Model file for the job. Use its own axes, mm. A direction names the side the tool comes from. Coordinates: 2 decimals unless noted, no trailing zeros. Write each loop counter-clockwise with the first axis right and the second up, starting at its lowest first coordinate (ties: lowest second). Pieces come first, ordered by that corner, then holes. Notation, with made-up numbers: M 40,7.5 L 91,7.5 A18 cw 91,24.5 Z; hole C 51.5,65.25 d8. An arc over 180 degrees is marked long. Put each result on its own line as item: value. Start each with the question number.
Q1. Drill centre lines: line 1 along Y through (x, z) = (0, 4.25); line 2 along X through (y, z) = (-0.5, 3.25); line 3 along Y through (x, z) = (60.5, 2.5). Where is each one in solid material? Low to high.
Q2. Cut at B-B (x = 0). Write the cut outline in (y, z), then the cut area to 3 significant figures.
Q3. Cut at C-C (y = -1.5). Write the cut outline in (x, z), then the cut area to 3 significant figures.
Q4. Cut at D-D (y = -13). Write the cut outline in (x, z), then the cut area to 3 significant figures.
Q5. Pull direction Y, two halves, no side cores. Call faces 4 (the flat face through (-10, 0, 4)), 5 (the cylindrical face through (65.302, -2.069, 3.698)), 6 (the flat face through (33, 10, 4)), 7 (the flat face through (28, -10, 4)): pulls with the +Y half, pulls with the -Y half, needs draft (parallel to the pull), parting line crosses it, or undercut.
Q6. Which spindle directions (+Z, -Z, +X, -X, +Y, -Y) get a long thin tool onto all of the face, cutting with end or side? Do faces 1 (the flat face through (33, -1, 7.5)), 2 (the cylindrical face through (73.07, -39.48, 9.19)), 3 (the flat face through (68, -25, 4)). Say none if no direction does.
Q7. Cut at A-A (z = 2.5). Write the cut outline in (x, y), then the cut area to 3 significant figures.
Q8. Drop flat-ended pins along their axis: pin 1 (2 mm diameter, centred on x = 59.5, z = 8, fed in from -Y); pin 2 (6 mm diameter, centred on y = -19, z = 8, fed in from -X); pin 3 (20 mm diameter, centred on x = 31, y = -10.5, fed in from +Z). Give the stop position or say it passes through.
```python
from build123d import *

# Parameters (mm, degrees)
SKETCH1_W           = 88
SKETCH1_H           = 20
SKETCH1_R           = 3.4
BOSS_EXTRUDE1_DEPTH = 7.5
SKETCH2_W           = 10
SKETCH2_H           = 7.5
BOSS_EXTRUDE2_DEPTH = 30
FILLET1_R           = 3


with BuildPart() as part:
    # Sketch1 → Boss-Extrude1 (new body)
    with BuildSketch(Plane.XY):
        with Locations((34, 0)):
            Rectangle(SKETCH1_W, SKETCH1_H)
        Circle(SKETCH1_R, mode=Mode.SUBTRACT)
        with Locations((68, 0)):
            Circle(SKETCH1_R, mode=Mode.SUBTRACT)
    extrude(amount=BOSS_EXTRUDE1_DEPTH)

    # Sketch2 → Boss-Extrude2 (add)
    with BuildSketch(Plane.XZ.offset(10)):
        with Locations((73, 3.75)):
            Rectangle(SKETCH2_W, SKETCH2_H)
    extrude(amount=BOSS_EXTRUDE2_DEPTH)

    # Sketch4 → Loft1 section 0
    with BuildSketch(Plane.XY.offset(7.5)):
        with BuildLine():
            Line((78, -40), (68, -40))
            Line((68, -40), (68, -30))
            Line((68, -30), (78, -30))
            Line((78, -30), (78, -40))
        make_face()
    # Sketch3 → Loft1 section 1
    with BuildSketch(Plane.XY.offset(10.5)):
        with BuildLine():
            Line((75.5, -35), (70.5, -35))
            Line((70.5, -35), (70.5, -40))
            Line((70.5, -40), (75.5, -40))
            Line((75.5, -40), (75.5, -35))
        make_face()
    loft()

    # Fillet1
    fillet1_edges = [part.edges().sort_by_distance(p)[0] for p in [
        (73, -35, 10.5),
        (75.5, -37.5, 10.5),
        (73, -40, 10.5),
        (70.5, -37.5, 10.5),
    ]]
    fillet(fillet1_edges, radius=FILLET1_R - 0.0001)  # a hair under: the kernel refuses the full size


solid = part.part
```
Computed values:
1. line 1: -10 to -3.4, 3.4 to 10
1. line 2: -10 to -3.36, 3.36 to 64.64, 71.36 to 78
1. line 3: -10 to 10
2. outline: M -10,0 L -3.4,0 L -3.4,7.5 L -10,7.5 Z; M 3.4,0 L 10,0 L 10,7.5 L 3.4,7.5 Z
2. area: 99.0 mm2
3. outline: M -10,0 L -3.05,0 L -3.05,7.5 L -10,7.5 Z; M 3.05,0 L 64.95,0 L 64.95,7.5 L 3.05,7.5 Z; M 71.05,0 L 78,0 L 78,7.5 L 71.05,7.5 Z
3. area: 568 mm2
4. outline: M 68,0 L 78,0 L 78,7.5 L 68,7.5 Z
4. area: 75.0 mm2
5. face 4: needs draft
5. face 5: undercut
5. face 6: pulls with the +Y half
5. face 7: pulls with the -Y half
6. face 1: +Z, +X, -X, +Y
6. face 2: +Z, +X, -X, -Y
6. face 3: +Z, -Z, -X, -Y
7. outline: M -10,-10 L 68,-10 L 68,-40 L 78,-40 L 78,10 L -10,10 Z; hole C 0,0 d6.8; hole C 68,0 d6.8
7. area: 1,990 mm2
8. pin 1: y = -10
8. pin 2: x = 68
8. pin 3: z = 7.5
